```python
from build123d import *

# Parameters (mm, degrees)
BOSS_EXTRUDE1_DEPTH = 10
SKETCH2_W           = 8
SKETCH2_H           = 20
CUT_EXTRUDE1_DEPTH  = 20
SKETCH3_W           = 8
SKETCH3_H           = 10
CUT_EXTRUDE2_DEPTH  = 34.541019662
SKETCH4_R           = 1.25
SKETCH4_R_2         = 2.5
CUT_EXTRUDE3_DEPTH  = 10


with BuildPart() as part:
    # Sketch1 → Boss-Extrude1 (new body)
    with BuildSketch(Plane.XY):
        Polygon((0, 0), (40, -15), (40, 25), (0, 25), align=None)
    extrude(amount=BOSS_EXTRUDE1_DEPTH)

    # Sketch2 → Cut-Extrude1 (cut)
    with BuildSketch(Plane.ZY):
        with Locations((5, 12)):
            Rectangle(SKETCH2_W, SKETCH2_H)
    extrude(amount=-CUT_EXTRUDE1_DEPTH, mode=Mode.SUBTRACT)

    # Sketch3 → Cut-Extrude2 (cut, through all)
    with BuildSketch(Plane.ZY.offset(-20)):
        with Locations((5, 7)):
            Rectangle(SKETCH3_W, SKETCH3_H)
    extrude(amount=-CUT_EXTRUDE2_DEPTH, mode=Mode.SUBTRACT)

    # Sketch4 → Cut-Extrude3 (cut)
    with BuildSketch(Plane.XY.offset(10)):
        with Locations((5, 18)):
            Circle(SKETCH4_R)
        with Locations((5, 8)):
            Circle(SKETCH4_R)
        with Locations((30, 20)):
            Circle(SKETCH4_R_2)
        with Locations((30, -5)):
            Circle(SKETCH4_R_2)
    extrude(amount=-CUT_EXTRUDE3_DEPTH, mode=Mode.SUBTRACT)


solid = part.part
```
Check sheet for the modelled part. Datum: model origin and axes. Units: mm. A direction names the side the tool comes from. Give positions to 0.01 mm unless a question says otherwise; leave off trailing zeros. Write each loop counter-clockwise with the first axis right and the second up, starting at its lowest first coordinate (ties: lowest second). Pieces come first, ordered by that corner, then holes. Notation, with made-up numbers: (47.25, 18.25) - (106.25, 18.25) arc R21 cw to (106.25, 41.25) - close; hole circle Ø4 at (69.5, -21). An arc over 180 degrees is marked (long way). Answer as a JSON object with one key per item and string values. Group by question number.
1) Sectioned sample at B-B (z = 1.5). Record the cut outline in (x, y).
2) Sectioned sample at A-A (x = 30). Record the cut outline in (y, z), then the cut area to 4 significant figures.
3) Sectioned sample at D-D (x = 16). Record the cut outline in (y, z).
4) Access from +Z, -Z, +X, -X, +Y, -Y to the whole of each face (thin tool, end or side, straight path). Record for faces 1 (the face through (10, 22, 5)), 2 (the face through (30, 12, 5)), 3 (the face through (0, 12.7, 9.4)).
5) Depth check by flat-ended pin: P1, Ø4, axis at x = 10.5, z = 7, coming from the -Y side; P2, Ø4, axis at x = 27, z = 5.5, coming from the -Y side (3 decimals); P3, Ø4, axis at x = 13.5, z = 5.5, coming from the -Y side. Enter the tip coordinate at first touch or a pass-through.
6) Thickness scan on probe 1 along Y at (x, z) = (5, 9.55) (3 decimals); probe 2 along Y at (x, z) = (30, 5); probe 3 along Z at (x, y) = (16.5, 12.5). Record the ranges inside material, lowest first. Write a range as from..to.
7) Release check for a two-part mould opening along X. For faces 4 (the face through (20, 17, 5)), 5 (the face through (15, 10, 9)), 6 (the face through (4.73, 6.78, 9.51)) record: pulls with the +X half, pulls with the -X half, needs draft (parallel to the pull), parting line crosses it, or undercut.
8) Sectioned sample at C-C (y = 18). Record the cut outline in (x, z).
Geometry results:
{
 "1": {"outline": "(0, 0) - (40, -15) - (40, 2) - (0, 2) - close; (0, 22) - (20, 22) - (20, 12) - (40, 12) - (40, 25) - (0, 25) - close; hole circle Ø5 at (30, -5); hole circle Ø5 at (30, 20)"},
 "2": {"outline": "(-11.25, 0) - (-7.5, 0) - (-7.5, 10) - (-11.25, 10) - close; (-2.5, 0) - (17.5, 0) - (17.5, 10) - (-2.5, 10) - close; (22.5, 0) - (25, 0) - (25, 10) - (22.5, 10) - close; hole (2, 1) - (12, 1) - (12, 9) - (2, 9) - close", "area": "182.5 mm^2"},
 "3": {"outline": "(-6, 0) - (25, 0) - (25, 10) - (-6, 10) - close; hole (2, 1) - (22, 1) - (22, 9) - (2, 9) - close"},
 "4": {"face 1": "-X", "face 2": "+X, -X", "face 3": "+Z, -Z, -X, +Y, -Y"},
 "5": {"P1": "stops at y = -4.69", "P2": "stops at y = -10.875", "P3": "stops at y = -5.81"},
 "6": {"probe 1": "y = -1.875..6.75, 9.25..16.75, 19.25..25", "probe 2": "y = -11.25..-7.5, -2.5..2, 12..17.5, 22.5..25", "probe 3": "z = 0..1, 9..10"},
 "7": {"face 4": "pulls with the -X half", "face 5": "needs draft", "face 6": "undercut"},
 "8": {"outline": "(0, 0) - (3.75, 0) - (3.75, 1) - (0, 1) - close; (0, 9) - (3.75, 9) - (3.75, 10) - (0, 10) - close; (6.25, 0) - (28.5, 0) - (28.5, 10) - (6.25, 10) - (6.25, 9) - (20, 9) - (20, 1) - (6.25, 1) - close; (31.5, 0) - (40, 0) - (40, 10) - (31.5, 10) - close"}
}
